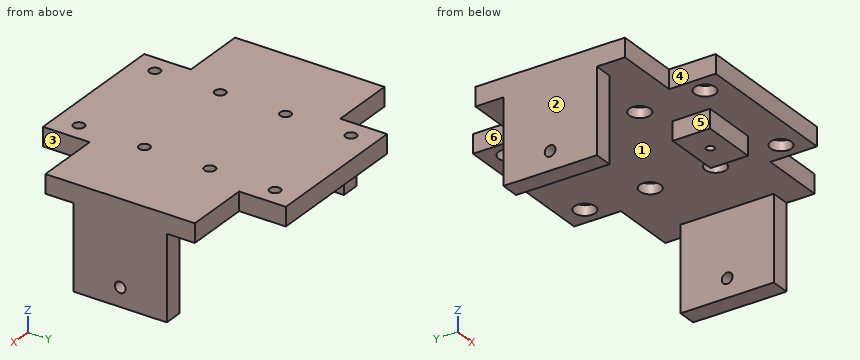
```python
from build123d import *

# Parameters (mm, degrees)
SKETCH043_W         = 150
SKETCH043_H         = 80
SKETCH043_W_2       = 80
SKETCH043_H_2       = 25
PAD021_DEPTH        = 10
HOLE020_D           = 5.8
HOLE020_DEPTH       = 25
HOLE020_CBORE_D     = 11.2
HOLE020_CBORE_DEPTH = 5.4
SKETCH044_W         = 10
SKETCH044_H         = 50
PAD022_DEPTH        = 45
SKETCH045_R         = 2.9
HOLE021_DEPTH       = 75.001
SKETCH046_R         = 2.9
HOLE022_DEPTH       = 75.001
SKETCH047_W         = 30
SKETCH047_H         = 20
PAD023_DEPTH        = 10
SKETCH048_R         = 2.1
HOLE023_DEPTH       = 45.001


with BuildPart() as part:
    # Sketch043 → Pad021 (new body)
    with BuildSketch(Plane.XY):
        Rectangle(SKETCH043_W, SKETCH043_H)
        with Locations((0, 52.5)):
            Rectangle(SKETCH043_W_2, SKETCH043_H_2)
        with Locations((0, -52.5)):
            Rectangle(SKETCH043_W_2, SKETCH043_H_2)
    extrude(amount=PAD021_DEPTH)

    # Hole020
    with Locations(Plane(origin=(0, 0, 0), x_dir=(1, 0, 0), z_dir=(0, 0, -1))):
        with Locations((-30, -52.5), (30, -52.5), (-30, -17.5), (30, -17.5), (-30, 17.5), (30, 17.5), (-30, 52.5), (30, 52.5)):
            CounterBoreHole(HOLE020_D / 2, HOLE020_CBORE_D / 2, HOLE020_CBORE_DEPTH, depth=HOLE020_DEPTH)

    # Sketch044 → Pad022 (join)
    with BuildSketch(Plane.XY):
        with Locations((-70, 0)):
            Rectangle(SKETCH044_W, SKETCH044_H)
        with Locations((70, 0)):
            Rectangle(SKETCH044_W, SKETCH044_H)
    extrude(amount=-PAD022_DEPTH)

    # Sketch045 → Hole021 (cut, through all)
    with BuildSketch(Plane.YZ):
        with Locations((0, -35)):
            Circle(SKETCH045_R)
    extrude(amount=-HOLE021_DEPTH, mode=Mode.SUBTRACT)

    # Sketch046 → Hole022 (cut, through all)
    with BuildSketch(Plane.YZ):
        with Locations((0, -35)):
            Circle(SKETCH046_R)
    extrude(amount=HOLE022_DEPTH, mode=Mode.SUBTRACT)

    # Sketch047 → Pad023 (join)
    with BuildSketch(Plane.XY):
        with Locations((0, -35)):
            Rectangle(SKETCH047_W, SKETCH047_H)
    extrude(amount=-PAD023_DEPTH)

    # Sketch048 → Hole023 (cut, through all)
    with BuildSketch(Plane.XY):
        with Locations((0, -35)):
            Circle(SKETCH048_R)
    extrude(amount=-HOLE023_DEPTH, mode=Mode.SUBTRACT)


solid = part.part
```
Part model, mm, in its own coordinate system. Face numbers are marked on the shaded views. A direction names the side the tool comes from. Give positions to 0.01 mm unless a question says otherwise; leave off trailing zeros. Order: outer loops, then holes, each group sorted by start corner. A loop starts at its lowest first (then second) coordinate and runs counter-clockwise, first axis right, second up. Notation, with made-up numbers: M 11,69 L 63,69 A26 cw 63,99 Z; hole C 54.25,87.25 d6. An arc over 180 degrees is marked long. Use a Markdown table: item, result. Add a question column.
(1) Mould opens along X. For the marked faces 1, 2 and 3 say: +X half, -X half, draft (parallel to the pull), parting line (faces both ways), or undercut.
(2) Saw through at A-A, the plane y = -17.5. Give the cut face in (x, z), and give its area (3 significant figures).
(3) 3-axis set-ups, long thin cutter, end or side, ignore diameter. For the marked faces 4, 5 and 6: which of +Z, -Z, +X, -X, +Y, -Y reach the whole face in a straight line?
(4) Saw through at C-C, the plane x = 0. Give the cut face in (y, z).
(5) Drop flat-ended pins along their axis: P1, Ø1.5, axis at x = 15, y = 9, coming from the -Z side; P2, Ø3.5, axis at x = 28, y = -15.5, coming from the -Z side; P3, Ø12, axis at x = -45, y = 48, coming from the +Z side; P4, Ø8, axis at y = -56.5, z = 7.5, coming from the -X side. Give the stop position or say it passes through.
(6) Probe line 1 along Y through (x, z) = (30, 1.8); line 2 along Y through (x, z) = (-30, 9); line 3 along X through (y, z) = (52.5, 8.85). List the from-to ranges inside material, lowest first. Write a range as [from, to].
(7) Saw through at D-D, the plane z = 3. Give the number of separate pieces and of enclosed holes in the cut face, and give its area (3 significant figures).
(8) Saw through at B-B, the plane z = -22. Give the cut face in (x, y).
Answer key:
| question | item | result |
|---|---|---|
| 1 | face 1 | undercut |
| 1 | face 2 | -X half |
| 1 | face 3 | +X half |
| 2 | outline | M -75,-45 L -65,-45 L -65,0 L -35.6,0 L -35.6,5.4 L -32.9,5.4 L -32.9,10 L -75,10 Z; M -27.1,5.4 L -24.4,5.4 L -24.4,0 L 24.4,0 L 24.4,5.4 L 27.1,5.4 L 27.1,10 L -27.1,10 Z; M 32.9,5.4 L 35.6,5.4 L 35.6,0 L 65,0 L 65,-45 L 75,-45 L 75,10 L 32.9,10 Z |
| 2 | area | 2,230 mm^2 |
| 3 | face 4 | +Z, -Z, -X, -Y |
| 3 | face 5 | -Z, -X, +Y, -Y |
| 3 | face 6 | +Z, -Z, -X, +Y |
| 4 | outline | M -65,0 L -45,0 L -45,-10 L -37.1,-10 L -37.1,0 L -32.9,0 L -32.9,-10 L -25,-10 L -25,0 L 65,0 L 65,10 L -65,10 Z |
| 5 | P1 | z = 0 |
| 5 | P2 | z = 5.4 |
| 5 | P3 | z = 10 |
| 5 | P4 | x = -40 |
| 6 | line 1 | [-65, -58.1], [-46.9, -23.1], [-11.9, 11.9], [23.1, 46.9], [58.1, 65] |
| 6 | line 2 | [-65, -55.4], [-49.6, -20.4], [-14.6, 14.6], [20.4, 49.6], [55.4, 65] |
| 6 | line 3 | [-40, -32.9], [-27.1, 27.1], [32.9, 40] |
| 7 | separate pieces | 1 |
| 7 | enclosed holes | 8 |
| 7 | area | 15,200 mm^2 |
| 8 | outline | M -75,-25 L -65,-25 L -65,25 L -75,25 Z; M 65,-25 L 75,-25 L 75,25 L 65,25 Z |
